Here's how the part is built. I have some questions about the finished solid (model axes, mm). A direction names the side the tool comes from. Give positions to 0.01 mm unless a question says otherwise; leave off trailing zeros. Write each loop counter-clockwise with the first axis right and the second up, starting at its lowest first coordinate (ties: lowest second). Pieces come first, ordered by that corner, then holes. Notation, with made-up numbers: (45.25, 58.25) - (83.25, 58.25) arc R29 cw to (83.25, 84.25) - close; hole circle Ø7 at (53.5, 68.5). An arc over 180 degrees is marked (long way). One line per item, written item: value. Start each with the question number.
1) Please list where these lines run through material, in increasing order: L1, parallel to X at y = -7, z = 8.25; L2, parallel to Y at x = -41, z = 14.75; L3, parallel to Y at x = -31.5, z = 9.5. Write a range as [from, to].
2) Imagine slicing it at A-A on z = 8. Write out the boundary of the cut face in (x, y).
3) Imagine slicing it at B-B on x = -34.5. Write out the boundary of the cut face in (y, z).
4) On a 3-axis mill with a long thin cutter (end or side, diameter ignored), from which of +Z, -Z, +X, -X, +Y, -Y can I reach the whole of each face in a straight line? I mean faces 4 (the flat face through (-64, 8.218, 7)), 5 (the flat face through (-39, 25.218, 7)), 6 (the flat face through (-66.457, -6, 7)), 7 (the flat face through (-34, 8.218, 7)). Say none if no direction works.
5) Imagine slicing it at D-D on x = -40.5. Write out the boundary of the cut face in (y, z), plus the area to 3 significant figures.
6) We'd pull the mould along X, two halves only. Please class faces 1 (the flat face through (-59, 25.218, 7)), 2 (the flat face through (-60.957, 24, 7)), 3 (the cylindrical face through (-42.095, 23.742, 7.395)): +X half, -X half, draft (parallel to the pull), parting line (faces both ways), or undercut.
7) I'm going to push flat-ended pins straight in: P1, Ø5, axis at x = -58.5, y = 3, coming from the -Z side; P2, Ø8, axis at y = 13, z = 3.5, coming from the +X side; P3, Ø3.5, axis at y = 24, z = 9.5, coming from the -X side; P4, Ø11, axis at x = -48.96, y = 17.22, coming from the -Z side. Where does each tip first touch, or does it pass through?
8) Imagine slicing it at C-C on y = 12. Write out the boundary of the cut face in (x, z), plus the area to 3 significant figures.
from build123d import *

# Parameters (mm, degrees)
CROQUIS1_W              = 35
CROQUIS1_H              = 22
SALIENTE_EXTRUIR1_DEPTH = 15


with BuildPart() as part:
    # Croquis1 → Saliente-Extruir1 (new body)
    with BuildSketch(Plane.XY):
        with BuildLine():
            Line((-69.45710358, 8.218313922), (-69.45710358, -19.781686078))
            Line((-69.45710358, -19.781686078), (-28.45710358, -19.781686078))
            Line((-28.45710358, -19.781686078), (-28.45710358, 8.218313922))
            Line((-28.45710358, 8.218313922), (-39.57627206, 8.218313922))
            ThreePointArc((-39.57627206, 8.218313922), (-36.178802084, 14.827705029), (-36.95710358, 22.218313922))
            Line((-36.95710358, 22.218313922), (-36.95710358, 25.218313922))
            Line((-36.95710358, 25.218313922), (-41.473788806, 25.218313922))
            ThreePointArc((-41.473788806, 25.218313922), (-42.09510915, 23.718313922), (-41.473788806, 22.218313922))
            ThreePointArc((-41.473788806, 22.218313922), (-48.95710358, 8.218313922), (-56.440418353, 22.218313922))
            ThreePointArc((-56.440418353, 22.218313922), (-55.81909801, 23.718313922), (-56.440418353, 25.218313922))
            Line((-56.440418353, 25.218313922), (-60.95710358, 25.218313922))
            Line((-60.95710358, 25.218313922), (-60.95710358, 22.218313922))
            ThreePointArc((-60.95710358, 22.218313922), (-61.735405076, 14.827705029), (-58.3379351, 8.218313922))
            Line((-58.3379351, 8.218313922), (-69.45710358, 8.218313922))
        make_face()
        with Locations((-48.95710358, -5.781686078)):
            Rectangle(CROQUIS1_W, CROQUIS1_H, mode=Mode.SUBTRACT)
    extrude(amount=SALIENTE_EXTRUIR1_DEPTH)


solid = part.part
Numbers:
1. L1: [-69.46, -66.46], [-31.46, -28.46]
1. L2: [-19.78, -16.78], [5.22, 13.01], [21.42, 25.22]
1. L3: [-19.78, -16.78], [5.22, 8.22]
2. outline: (-69.46, -19.78) - (-28.46, -19.78) - (-28.46, 8.22) - (-39.58, 8.22) arc R13 ccw to (-36.96, 22.22) - (-36.96, 25.22) - (-41.47, 25.22) arc R2.12 ccw to (-41.47, 22.22) arc R9 cw (long way) to (-56.44, 22.22) arc R2.12 ccw to (-56.44, 25.22) - (-60.96, 25.22) - (-60.96, 22.22) arc R13 ccw to (-58.34, 8.22) - (-69.46, 8.22) - close; hole (-66.46, -16.78) - (-31.46, -16.78) - (-31.46, 5.22) - (-66.46, 5.22) - close
3. outline: (-19.78, 0) - (-16.78, 0) - (-16.78, 15) - (-19.78, 15) - close; (5.22, 0) - (8.22, 0) - (8.22, 15) - (5.22, 15) - close
4. face 4: +Z, -Z, -X
4. face 5: +Z, -Z, +X, -X, +Y
4. face 6: +Z, -Z
4. face 7: +Z, -Z, +X
5. outline: (-19.78, 0) - (-16.78, 0) - (-16.78, 15) - (-19.78, 15) - close; (5.22, 0) - (14.14, 0) - (14.14, 15) - (5.22, 15) - close; (20.3, 0) - (25.22, 0) - (25.22, 15) - (20.3, 15) - close
5. area: 253 mm^2
6. face 1: draft
6. face 2: -X half
6. face 3: undercut
7. P1: z = 0
7. P2: x = -35.96
7. P3: x = -60.96
7. P4: through
8. outline: (-60.86, 0) - (-56.29, 0) - (-56.29, 15) - (-60.86, 15) - close; (-41.62, 0) - (-37.05, 0) - (-37.05, 15) - (-41.62, 15) - close
8. area: 137 mm^2
